Check sheet for the modelled part. Datum: model origin and axes. Units: mm. A direction names the side the tool comes from. Round coordinates to 2 decimals unless told otherwise and drop trailing zeros. Order: outer loops, then holes, each group sorted by start corner. A loop starts at its lowest first (then second) coordinate and runs counter-clockwise, first axis right, second up. Notation, with made-up numbers: M 45,8.25 L 93,8.25 A12 cw 93,21.25 Z; hole C -15,-6 d10. An arc over 180 degrees is marked long. One line per item, written item: value. Start each with the question number.
(1) Depth check by flat-ended pin: pin 1 Ø1.5 at (x, z) = (11, -1) entering from +Y; pin 2 Ø1 at (x, z) = (55, 0) entering from -Y; pin 3 Ø3 at (y, z) = (10, -1) entering from -X. Enter the tip coordinate at first touch or a pass-through.
(2) Access from +Z, -Z, +X, -X, +Y, -Y to the whole of each face (thin tool, end or side, straight path). Record for faces 1 (the face through (-13.786, 0.216, -0.042)), 2 (the face through (-12.986, 0.203, -0.042)).
(3) Cross-section at B-B, the plane y = 0. Enter the section's corners in (x, z).
(4) Cross-section at C-C, the plane z = -0.1. Enter the section's corners in (x, y), and give its area (3 significant figures).
(5) Thickness scan on L1, parallel to Y at x = 47.89, z = 0.7; L2, parallel to X at y = 0, z = -0.6; L3, parallel to Y at x = 11.5, z = -1.95. Record the ranges inside material, lowest first.
(6) Cross-section at A-A, the plane x = 47.89. Enter the section's corners in (y, z), and give its area (3 significant figures).
from build123d import *

# Parameters (mm, degrees)
EXTRUDE_1_DEPTH      = 3
EXTRUDE_1_DEPTH_BACK = 3


with BuildPart() as part:
    # 草图1 → 凸台-拉伸1 (new, two sides: drawn at the far end of the back side and taken through both)
    with BuildSketch(Plane.XY.offset(-EXTRUDE_1_DEPTH_BACK)):
        with BuildLine():
            Line((-6.048545797, -12.390498432), (32.625436737, -31.269590002))
            ThreePointArc((32.625436737, -31.269590002), (82.6864675, 0), (32.625436737, 31.269590002))
            Line((32.625436737, 31.269590002), (-6.048545797, 12.390498432))
            ThreePointArc((-6.048545797, 12.390498432), (-13.788015, 0), (-6.048545797, -12.390498432))
        make_face()
        with BuildLine():
            Line((-5.697600672, -11.671584306), (32.976381862, -30.550675876))
            ThreePointArc((32.976381862, -30.550675876), (81.8864675, 0), (32.976381862, 30.550675876))
            Line((32.976381862, 30.550675876), (-5.697600672, 11.671584306))
            ThreePointArc((-5.697600672, 11.671584306), (-12.988015, 0), (-5.697600672, -11.671584306))
        make_face(mode=Mode.SUBTRACT)
    extrude(amount=EXTRUDE_1_DEPTH + EXTRUDE_1_DEPTH_BACK)


solid = part.part
Values found:
1. pin 1: y = 21.08
1. pin 2: y = -34.16
1. pin 3: x = -10.86
2. face 1: +Z, -Z, -X
2. face 2: +Z, -Z
3. outline: M -13.79,-3 L -12.99,-3 L -12.99,3 L -13.79,3 Z; M 81.89,-3 L 82.69,-3 L 82.69,3 L 81.89,3 Z
4. outline: M -6.05,-12.39 L 32.63,-31.27 A34.8 ccw long 32.63,31.27 L -6.05,12.39 A13.79 ccw Z; hole M -5.7,-11.67 L 32.98,-30.55 A34 ccw long 32.98,30.55 L -5.7,11.67 A12.99 ccw Z
4. area: 204 mm^2
5. L1: -34.8 to -34, 34 to 34.8
5. L2: -13.79 to -12.99, 81.89 to 82.69
5. L3: -20.96 to -20.07, 20.07 to 20.96
6. outline: M -34.8,-3 L -34,-3 L -34,3 L -34.8,3 Z; M 34,-3 L 34.8,-3 L 34.8,3 L 34,3 Z
6. area: 9.60 mm^2
